Check sheet for the modelled part. Datum: model origin and axes. Units: mm. A direction names the side the tool comes from. Coordinates: 2 decimals unless noted, no trailing zeros. Write each loop counter-clockwise with the first axis right and the second up, starting at its lowest first coordinate (ties: lowest second). Pieces come first, ordered by that corner, then holes. Notation, with made-up numbers: (23.25, 34.25) -> (73.25, 34.25) arc R21 cw to (73.25, 39.25) -> close; hole circle Ø7 at (80, -12.75). An arc over 180 degrees is marked (long way). Put each result on its own line as item: value.
```python
from build123d import *

# Parameters (mm, degrees)
F0_R           = 10
F1_DEPTH       = 20
F2_SIZE        = 1
F4_D           = 5.4
F4_CBORE_D     = 11
F4_CBORE_DEPTH = 5.8


with BuildPart() as f1:
    # F0 (on Top) → F1 (new body)
    with BuildSketch(Plane.XY):
        with Locations((-63.557699, 20.238634)):
            Circle(F0_R)
    extrude(amount=F1_DEPTH)

    # F2
    f2_edges = [f1.edges().sort_by_distance(p)[0] for p in [
        (-73.557699, 20.238634, 20),
    ]]
    chamfer(f2_edges, length=F2_SIZE)

    # F4 (through all)
    with Locations(Plane.XY.offset(20)):
        with Locations((-63.557699, 20.238634)):
            CounterBoreHole(F4_D / 2, F4_CBORE_D / 2, F4_CBORE_DEPTH)


solid = f1.part
```
Q1. Cross-section at A-A (z = 17). Record the cut outline in (x, y).
Recorded:
outline: circle Ø20 at (-63.56, 20.24); hole circle Ø11 at (-63.56, 20.24)
Q2. Material ranges on line 1 along Y through (x, z) = (-63.75, 11.5); line 2 along X through (y, z) = (20.25, 10); line 3 along Y through (x, z) = (-63, 8.25), recorded low to high.
Recorded:
line 1: y = 10.24 to 17.55, 22.93 to 30.24
line 2: x = -73.56 to -66.26, -60.86 to -53.56
line 3: y = 10.25 to 17.6, 22.88 to 30.22
Q3. Cross-section at B-B (z = 10.5). Record the cut outline in (x, y), plus the area to 3 significant figures.
Recorded:
outline: circle Ø20 at (-63.56, 20.24); hole circle Ø5.4 at (-63.56, 20.24)
area: 291 mm2
Q4. Mould release check, pull along Y, two halves, no side actions. Record for faces 1 (the cylindrical face through (-65.009, 22.515, 7.001)), 2 (the cylindrical face through (-67.92, 16.89, 17.14)), 3 (the cylindrical face through (-73.548, 20.678, 9.367)), 4 (the flat face through (-68, 16, 20)): released by +Y, released by -Y, zero draft, split by the parting line, or undercut.
Recorded:
face 1: undercut
face 2: undercut
face 3: split by the parting line
face 4: zero draft
Q5. Depth check by flat-ended pin: P1, Ø3, axis at y = 17, z = 9, coming from the +X side; P2, Ø12, axis at x = -62.5, y = 22.5, coming from the +Z side; P3, Ø2, axis at x = -69.5, z = 5.5, coming from the +Y side; P4, Ø12, axis at x = -57, z = 16, coming from the -Y side. Enter the tip coordinate at first touch or a pass-through.
Recorded:
P1: stops at x = -53.71
P2: stops at z = 20
P3: stops at y = 28.93
P4: stops at y = 10.25
Q6. Tool access check on faces 5 (the flat face through (-61, 18, 0)), 6 (the flat face through (-61, 22, 14.2)). Record the directions out of +Z, -Z, +X, -X, +Y, -Y that give a thin tool (end or side, any length) a straight path to the whole face; none if there is none.
Recorded:
face 5: -Z, +X, -X, +Y, -Y
face 6: +Z
